For this review, take the finished solid that the model builds, in its own axes (mm). A direction names the side the tool comes from. Give positions to 0.01 mm unless a question says otherwise; leave off trailing zeros. Order: outer loops, then holes, each group sorted by start corner. A loop starts at its lowest first (then second) coordinate and runs counter-clockwise, first axis right, second up. Notation, with made-up numbers: (84, 48.25) - (98, 48.25) arc R15 cw to (98, 65.25) - close; hole circle Ø2 at (-38.5, 70.25). An arc over 180 degrees is marked (long way). One line per item, written item: value.
```python
from build123d import *

# Parameters (mm, degrees)
F0_W     = 300
F0_H     = 300
F1_DEPTH = 200
F2_W     = 300
F2_H     = 200
F3_DEPTH = 50
F4_W     = 300
F4_H     = 200
F5_DEPTH = 50
F6_W     = 300
F6_H     = 200
F7_DEPTH = 50


with BuildPart() as f1:
    # F0 (on Top) → F1 (new body)
    with BuildSketch(Plane.XY):
        with Locations((6.017694, -6.54919)):
            Rectangle(F0_W, F0_H)
    extrude(amount=F1_DEPTH)

    # F2 (on face) → F3 (join)
    with BuildSketch(Plane.YZ.offset(156.017694)):
        with Locations((-6.54919, 100)):
            Rectangle(F2_W, F2_H)
    extrude(amount=F3_DEPTH)

    # F4 (on face) → F5 (join)
    with BuildSketch(Plane.XZ.offset(156.54919)):
        with Locations((56.017694, 100)):
            Rectangle(F4_W, F4_H)
    extrude(amount=F5_DEPTH)

    # F6 (on face) → F7 (join)
    with BuildSketch(Plane(origin=(0, 143.45081, 0), x_dir=(-1, 0, 0), z_dir=(0, 1, 0))):
        with Locations((-56.017694, 100)):
            Rectangle(F6_W, F6_H)
    extrude(amount=F7_DEPTH)


solid = f1.part
```
(1) Take a section at A-A (z = 13). Write out the cut boundary in (x, y).
Answers below:
outline: (-143.98, -156.55) - (-93.98, -156.55) - (-93.98, -206.55) - (206.02, -206.55) - (206.02, 193.45) - (-93.98, 193.45) - (-93.98, 143.45) - (-143.98, 143.45) - close
(2) For P1, Ø25, axis at y = -182, z = 112.5, coming from the -X side; P2, Ø5, axis at x = 19, y = 75.5, coming from the -Z side; P3, Ø15, axis at x = -116.5, z = 122, coming from the +Y side; P4, Ø15, axis at x = -117.5, z = 56, coming from the -Y side, all flat-tipped, find the tip position at first contact; note any pin that passes through.
Answers below:
P1: stops at x = -93.98
P2: stops at z = 0
P3: stops at y = 143.45
P4: stops at y = -156.55
(3) Wall thickness on line 1 (X direction, y = 160, z = 122); line 2 (Y direction, x = -99, z = 33.5): over which ranges is each line inside the solid? List them lowest first. Write a range as from..to.
Answers below:
line 1: x = -93.98..206.02
line 2: y = -156.55..143.45
(4) Take a section at B-B (y = 169.5). Write out the cut boundary in (x, z), then the cut area to 3 significant figures.
Answers below:
outline: (-93.98, 0) - (206.02, 0) - (206.02, 200) - (-93.98, 200) - close
area: 60,000 mm^2
(5) Machinability: for faces 1 (the face through (-93.982, 168, 99)), 2 (the face through (-119, -156.549, 99)), 3 (the face through (206.018, -9, 99)), which of the approach directions +Z, -Z, +X, -X, +Y, -Y give a long, thin tool a straight path to every point of the face, cutting with its end or side? Answer none if there is none.
Answers below:
face 1: +Z, -Z, -X, +Y
face 2: +Z, -Z, -X, -Y
face 3: +Z, -Z, +X, +Y, -Y
